from build123d import *

# Parameters (mm, degrees)
CUT_EXTRUDE1_DEPTH = 121


with BuildPart() as part:
    # Sketch1 → Revolve1 (revolve)
    with BuildSketch(Plane(origin=(0, 0, 0), x_dir=(0, 0, -1), z_dir=(1, 0, 0))):
        Polygon((10, 0), (80, 0), (80, 5), (75, 5), (75, 15), (80, 15), (80, 25), (75, 25), (75, 35), (80, 35), (80, 40), (10, 40), align=None)
    revolve(axis=Axis((0, 0, 0), (0, 1, 0)))

    # Sketch2 → Cut-Extrude1 (cut, through all)
    with BuildSketch(Plane.XZ):
        with BuildLine():
            Line((-4, 16.756133146), (4, 16.756133146))
            Line((4, 16.756133146), (4, 12.756133146))
            ThreePointArc((4, 12.756133146), (0, -13.36858006), (-4, 12.756133146))
            Line((-4, 12.756133146), (-4, 16.756133146))
        make_face()
    extrude(amount=-CUT_EXTRUDE1_DEPTH, mode=Mode.SUBTRACT)


solid = part.part
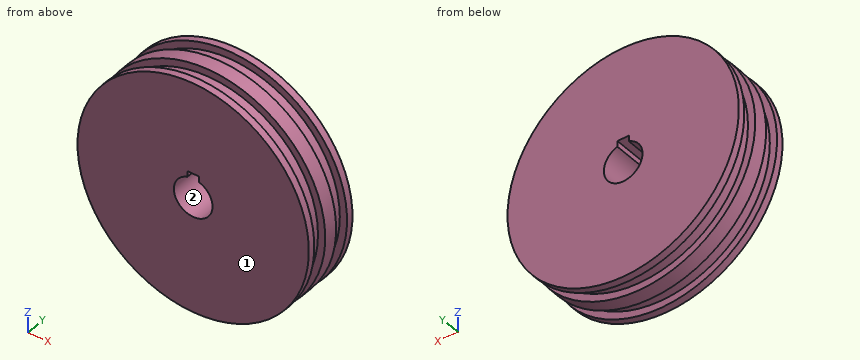
The model under review builds one solid part; all positions refer to its coordinate system, in mm. Face numbers are marked on the shaded views. Round coordinates to 2 decimals unless told otherwise and drop trailing zeros. Write each loop counter-clockwise with the first axis right and the second up, starting at its lowest first coordinate (ties: lowest second). Pieces come first, ordered by that corner, then holes. Notation, with made-up numbers: M 78.5,-19.75 L 105.5,-19.75 A20 ccw 105.5,15.25 Z; hole C 66.25,52 d1. An arc over 180 degrees is marked long. Use a Markdown table: item, result. Add a question column.
Q1. We need section D-D, the plane z = 19. State the section outline as (x, y) points.
Q2. Insertion check: pin 1 (5 mm diameter, centred on x = -18.5, y = 33, fed in from +Z); pin 2 (1.5 mm diameter, centred on x = -8.5, y = 32, fed in from +Z); pin 3 (12 mm diameter, centred on x = 29.5, z = 45, fed in from -Y); pin 4 (12 mm diameter, centred on y = 26.5, z = 28, fed in from +X). Each pin has a flat end and moves straight along its axis. Give the tip position at first contact, or say it passes through.
Q3. We need section C-C, the plane y = 9.5. State the section outline as (x, z) points.
Q4. We need section B-B, the plane z = 0. State the section outline as (x, y) points.
Q5. To check wall thickness, follow line 1 (Y direction, x = -64.5, z = 42.5); line 2 (X direction, y = 30.5, z = 0); line 3 (X direction, y = 28.5, z = 4). State the ranges of each line that lie inside material, in increasing order.
Q6. We need section A-A, the plane x = 0. State the section outline as (y, z) points.
Q7. The part is to be moulded in two halves that separate along X. For the marked faces 1 and 2, say which applies: pulls with the +X half, pulls with the -X half, needs draft (parallel to the pull), parting line crosses it, or undercut.
Findings below:
| question | item | result |
|---|---|---|
| 1 | outline | M -77.71,0 L 77.71,0 L 77.71,5 L 72.55,5 L 72.55,15 L 77.71,15 L 77.71,25 L 72.55,25 L 72.55,35 L 77.71,35 L 77.71,40 L -77.71,40 L -77.71,35 L -72.55,35 L -72.55,25 L -77.71,25 L -77.71,15 L -72.55,15 L -72.55,5 L -77.71,5 Z |
| 2 | pin 1 | stops at z = 78.17 |
| 2 | pin 2 | stops at z = 74.6 |
| 2 | pin 3 | stops at y = 0 |
| 2 | pin 4 | stops at x = 76.86 |
| 3 | outline | C 0,0 d150; hole M -4,12.76 A13.37 ccw long 4,12.76 L 4,16.76 L -4,16.76 Z |
| 4 | outline | M -80,0 L -13.37,0 L -13.37,40 L -80,40 L -80,35 L -75,35 L -75,25 L -80,25 L -80,15 L -75,15 L -75,5 L -80,5 Z; M 13.37,0 L 80,0 L 80,5 L 75,5 L 75,15 L 80,15 L 80,25 L 75,25 L 75,35 L 80,35 L 80,40 L 13.37,40 Z |
| 5 | line 1 | y = 0 to 5, 15 to 25, 35 to 40 |
| 5 | line 2 | x = -75 to -13.37, 13.37 to 75 |
| 5 | line 3 | x = -74.89 to -12.76, 12.76 to 74.89 |
| 6 | outline | M 0,-80 L 5,-80 L 5,-75 L 15,-75 L 15,-80 L 25,-80 L 25,-75 L 35,-75 L 35,-80 L 40,-80 L 40,-13.37 L 0,-13.37 Z; M 0,16.76 L 40,16.76 L 40,80 L 35,80 L 35,75 L 25,75 L 25,80 L 15,80 L 15,75 L 5,75 L 5,80 L 0,80 Z |
| 7 | face 1 | needs draft |
| 7 | face 2 | undercut |
